Check sheet for the drawn part. Datum: minimum x, y, z corner. Units: mm. A direction names the side the tool comes from. Coordinates: 2 decimals unless noted, no trailing zeros. Write each loop counter-clockwise with the first axis right and the second up, starting at its lowest first coordinate (ties: lowest second). Pieces come first, ordered by that corner, then holes. Notation, with made-up numbers: (-5.75, 78.5) -> (48.25, 78.5) arc R34 ccw to (48.25, 117.5) -> close; hole circle Ø11 at (83.5, 6.25). An arc over 180 degrees is marked (long way). One line per question, with ' | ' between items.
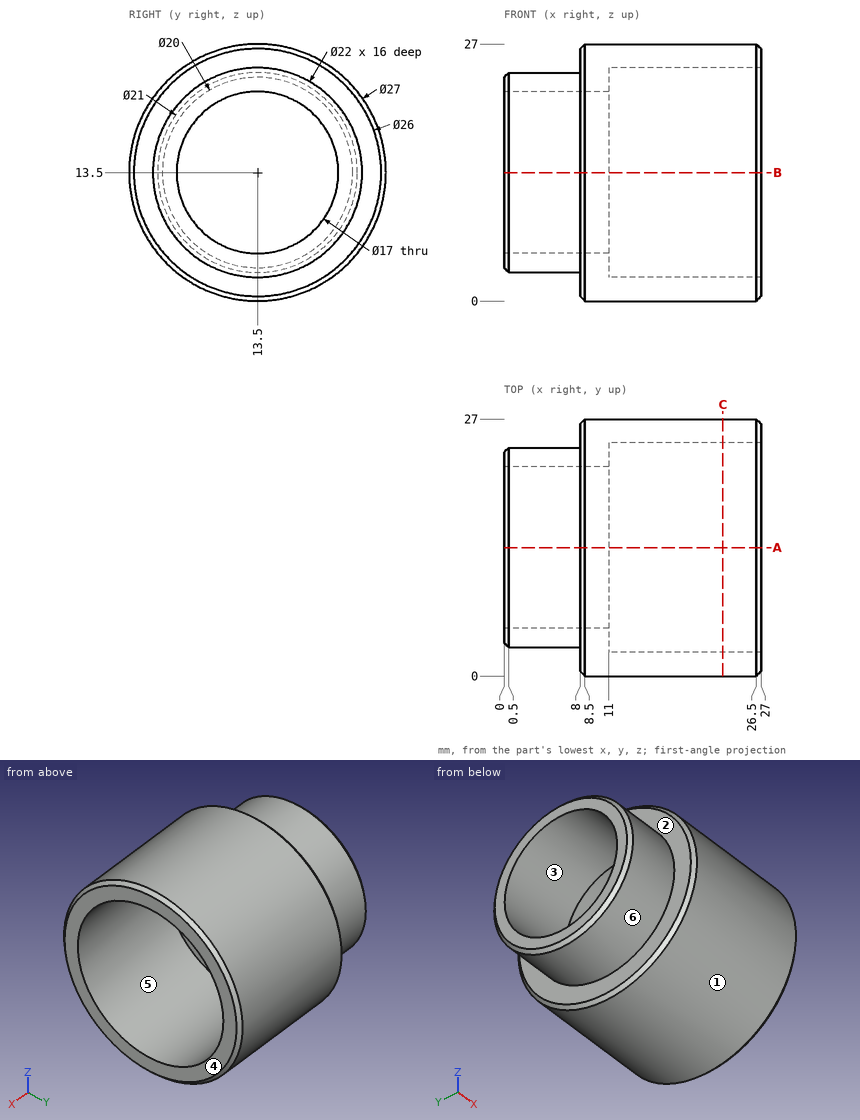
1. Mould release check, pull along Y, two halves, no side actions. Record for the marked faces 1, 2 and 3: released by +Y, released by -Y, zero draft, split by the parting line, or undercut.
Worked answers:
face 1: split by the parting line | face 2: zero draft | face 3: undercut
2. Cross-section at A-A on y = 13.5. Record the boundary of the cut face in (x, z).
Worked answers:
outline: (0, 3.5) -> (0.5, 3) -> (8, 3) -> (8, 0.5) -> (8.5, 0) -> (26.5, 0) -> (27, 0.5) -> (27, 2.5) -> (11, 2.5) -> (11, 5) -> (0, 5) -> close; (0, 22) -> (11, 22) -> (11, 24.5) -> (27, 24.5) -> (27, 26.5) -> (26.5, 27) -> (8.5, 27) -> (8, 26.5) -> (8, 24) -> (0.5, 24) -> (0, 23.5) -> close
3. Tool access check on the marked faces 4, 5 and 6. Record the directions out of +Z, -Z, +X, -X, +Y, -Y that give a thin tool (end or side, any length) a straight path to the whole face; none if there is none.
Worked answers:
face 4: +Z, -Z, +X, +Y, -Y | face 5: +X | face 6: -X
4. Cross-section at C-C on x = 23. Record the boundary of the cut face in (y, z), and give its area (3 significant figures).
Worked answers:
outline: circle Ø27 at (13.5, 13.5); hole circle Ø22 at (13.5, 13.5) | area: 192 mm²
5. Material ranges on line 1 (Z direction, x = 7.25, y = 13.5); line 2 (Z direction, x = 8.75, y = 13.5); line 3 (X direction, y = 22, z = 16.25), recorded low to high. Write a range as from..to.
Worked answers:
line 1: 3..5, 22..24 | line 2: 0..5, 22..27 | line 3: 0..11
6. Go/stop test with flat-tipped pins: P1, Ø8, axis at x = 16, y = 21.5, coming from the -Z side; P2, Ø5, axis at x = 7.5, y = 15, coming from the -Z side; P3, Ø5, axis at x = 20.5, y = 22, coming from the +Z side; P4, Ø1, axis at x = 15, y = 16.5, coming from the +Z side. Record where each tip stops, or that it passes through.
Worked answers:
P1: z = 0.61 | P2: z = 0 | P3: z = 25.59 | P4: z = 26.77
